Input: part model. Units: mm. Frame: model coordinates. Face numbers are marked on the shaded views. Give positions to 0.01 mm unless a question says otherwise; leave off trailing zeros. Write each loop counter-clockwise with the first axis right and the second up, starting at its lowest first coordinate (ties: lowest second). Pieces come first, ordered by that corner, then holes.
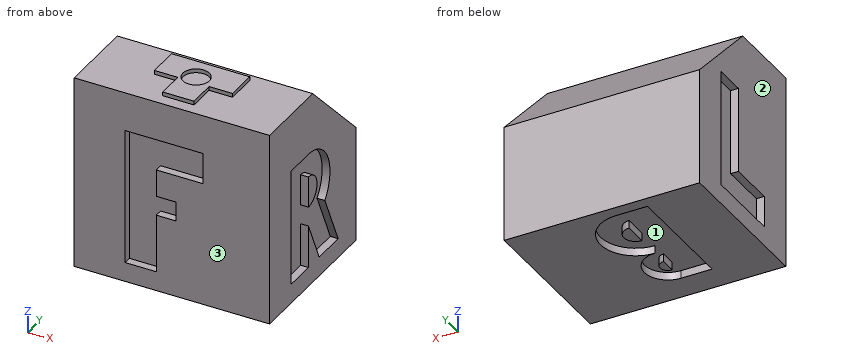
```python
from build123d import *

# Parameters (mm, degrees)
F0_W      = 50
F0_H      = 50
F1_DEPTH  = 40
F2_SIZE   = 20
F4_DEPTH  = 2
F6_DEPTH  = 2
F8_DEPTH  = 2
F9_R      = 3.387278
F10_DEPTH = 1
F12_DEPTH = 2


with BuildPart() as f1:
    # F0 (on Front) → F1 (new body)
    with BuildSketch(Plane.XZ):
        with Locations((-25, 25)):
            Rectangle(F0_W, F0_H)
    extrude(amount=-F1_DEPTH)

    # F2
    f2_edges = [f1.edges().sort_by_distance(p)[0] for p in [
        (-25, 40, 50),
    ]]
    chamfer(f2_edges, length=F2_SIZE)

    # F3 (on face) → F4 (cut)
    with BuildSketch(Plane.XZ):
        Polygon((-37, 40), (-37, 5), (-29, 5), (-29, 20), (-24, 20), (-24, 25), (-29, 25), (-29, 32), (-17, 32), (-17, 40), align=None)
    extrude(amount=-F4_DEPTH, mode=Mode.SUBTRACT)

    # F5 (on face) → F6 (cut)
    with BuildSketch(Plane.YZ):
        with BuildLine():
            Line((10, 35), (10, 5))
            Line((10, 5), (18, 5))
            Line((18, 5), (18, 16))
            Line((18, 16), (23, 5))
            Line((23, 5), (31.78767, 5))
            Line((31.78767, 5), (25.633212, 18.539808))
            ThreePointArc((25.633212, 18.539808), (27.071988, 29.207023), (18, 35))
            Line((18, 35), (10, 35))
        make_face()
        with BuildLine():
            Line((18, 21), (18, 29))
            ThreePointArc((18, 29), (22, 25), (18, 21))
        make_face(mode=Mode.SUBTRACT)
    extrude(amount=-F6_DEPTH, mode=Mode.SUBTRACT)

    # F7 (on face) → F8 (cut)
    with BuildSketch(Plane(origin=(-50, 0, 0), x_dir=(0, -1, 0), z_dir=(-1, 0, 0))):
        Polygon((-22, 35), (-30, 35), (-30, 5), (-10, 5), (-10, 13), (-22, 13), align=None)
    extrude(amount=-F8_DEPTH, mode=Mode.SUBTRACT)

    # F9 (on face) → F10 (join)
    with BuildSketch(Plane.XY.offset(50)):
        Polygon((-29, 10), (-29, 3), (-21, 3), (-21, 10), (-15, 10), (-15, 18), (-35, 18), (-35, 10), align=None)
        with Locations((-25.483249, 12.10618)):
            Circle(F9_R, mode=Mode.SUBTRACT)
    extrude(amount=F10_DEPTH)

    # F11 (on face) → F12 (cut)
    with BuildSketch(Plane(origin=(0, 0, 0), x_dir=(1, 0, 0), z_dir=(0, 0, -1))):
        with BuildLine():
            Line((-35, -7), (-35, -37))
            Line((-35, -37), (-27, -37))
            ThreePointArc((-27, -37), (-18, -28), (-27, -19))
            ThreePointArc((-27, -19), (-21, -13), (-27, -7))
            Line((-27, -7), (-35, -7))
        make_face()
        with BuildLine():
            ThreePointArc((-27, -25), (-24, -28), (-27, -31))
            Line((-27, -31), (-27, -25))
        make_face(mode=Mode.SUBTRACT)
        with BuildLine():
            Line((-27, -15), (-27, -11))
            ThreePointArc((-27, -11), (-25, -13), (-27, -15))
        make_face(mode=Mode.SUBTRACT)
    extrude(amount=-F12_DEPTH, mode=Mode.SUBTRACT)


solid = f1.part
```
Item 1: Section A-A (x = -36). Return loops of the section in (y, z), and give its area (3 significant figures).
Item 2: Section D-D (x = -11.5). Return loops of the section in (y, z), and give its area (3 significant figures).
Item 3: Section B-B (z = 37.5). Return loops of the section in (x, y), and give its area (4 significant figures).
Item 4: Pin query (flat end, axial travel): pin 1 (1 mm diameter, centred on x = -14, z = 33.5, fed in from +Y); pin 2 (6 mm diameter, centred on x = -25.48, y = 12.11, fed in from +Z); pin 3 (2 mm diameter, centred on x = -0.5, y = 25.5, fed in from +Z). Return the tip coordinate at first contact, or that it passes through.
Item 5: Mould query, pull axis X, two halves, no side actions, for the marked faces 1, 2 and 3. Classes: +X half, -X half, draft (parallel to the pull), parting line (faces both ways), or undercut.
Item 6: Ray query, line 1 (X direction, y = 24, z = 15.5); line 2 (Z direction, x = -38, y = 38); line 3 (Z direction, x = -33, y = 8). Return the intervals inside material, ascending.
Item 7: Section C-C (y = 4). Return loops of the section in (x, z), and give its area (3 significant figures).
Solved:
1. outline: (0, 0) - (40, 0) - (40, 30) - (20, 50) - (0, 50) - (0, 40) - (2, 40) - (2, 5) - (0, 5) - close
1. area: 1,730 mm2
2. outline: (0, 0) - (40, 0) - (40, 30) - (20, 50) - (0, 50) - close
2. area: 1,800 mm2
3. outline: (-50, 0) - (-37, 0) - (-37, 2) - (-17, 2) - (-17, 0) - (0, 0) - (0, 32.5) - (-50, 32.5) - close
3. area: 1,585 mm2
4. pin 1: stops at y = 37
4. pin 2: stops at z = 50
4. pin 3: stops at z = 45.5
5. face 1: undercut
5. face 2: -X half
5. face 3: draft
6. line 1: x = -48 to -2
6. line 2: z = 0 to 32
6. line 3: z = 2 to 50
7. outline: (-50, 0) - (0, 0) - (0, 50) - (-21, 50) - (-21, 51) - (-29, 51) - (-29, 50) - (-50, 50) - close
7. area: 2,510 mm2
